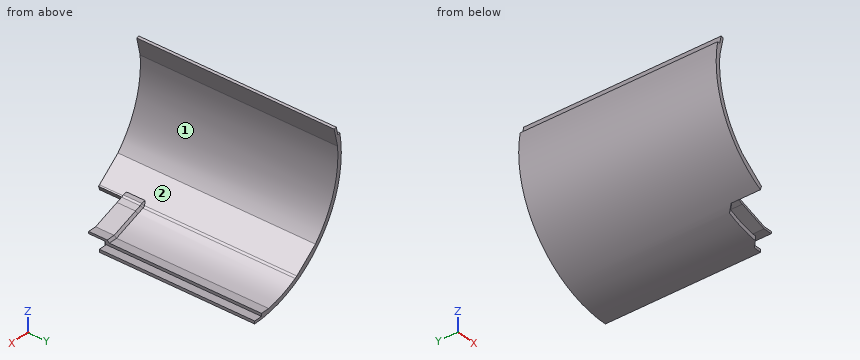
from build123d import *

# Parameters (mm, degrees)
EXTRUDE_1_DEPTH     = 96
CUT_EXTRUDE_1_DEPTH = 115.435602569
CUT_EXTRUDE_2_DEPTH = 125.800902391
EXTRUDE_2_DEPTH     = 10
CHAMFER_1_SIZE      = 1


with BuildPart() as part:
    # Эскиз1 → Бобышка-Вытянуть1 (new body)
    with BuildSketch(Plane(origin=(0, 0, 0), x_dir=(1, 0, 0), z_dir=(0, 1, 0))):
        with BuildLine():
            Line((-46.843090279, -12.726935731), (-48.838961005, -3.96936871))
            ThreePointArc((-48.838961005, -3.96936871), (-46.263287314, 16.146462365), (-35.762915695, 33.496475352))
            Line((-35.762915695, 33.496475352), (-24.862084305, 42.224125379))
            ThreePointArc((-24.862084305, 42.224125379), (-24.343954807, 42.524955783), (-23.822185811, 42.819428571))
            ThreePointArc((-23.822185811, 42.819428571), (-16.269960049, 46.22), (-8.252878286, 48.3))
            Line((-8.252878286, 48.3), (-4, 48.3))
            Line((-4, 48.3), (-4, 49.65))
            Line((-4, 49.65), (0, 49.65))
            Line((0, 49.65), (0, 51))
            ThreePointArc((0, 51), (-39.236846594, 32.580206711), (-50.131159715, -9.373730613))
            Line((-50.131159715, -9.373730613), (-48.950659721, -9.104691807))
            Line((-48.950659721, -9.104691807), (-48.061840279, -13.004691807))
            Line((-48.061840279, -13.004691807), (-46.843090279, -12.726935731))
        make_face()
    extrude(amount=EXTRUDE_1_DEPTH)

    # Эскиз2 → Вырез-Вытянуть1 (cut, through all)
    with BuildSketch(Plane(origin=(-12.717132038, 0, -36.127061224), x_dir=(0.9432653061224487, 0, -0.33204000100247416), z_dir=(0.33204000100247416, 0, 0.9432653061224487))):
        Polygon((8.752878286, 0), (8.752878286, 17.5), (-5.459985067, 17.5), (-8.752878286, 14.207106781), (-8.752878286, 0), (-8.252878286, 0), (8.252878286, 0), align=None)
    extrude(amount=-CUT_EXTRUDE_1_DEPTH, mode=Mode.SUBTRACT)

    # Эскиз3 → Вырез-Вытянуть2 (cut, through all)
    with BuildSketch(Plane.XY.offset(-48.3)):
        Polygon((-3.5, 20), (0, 20), (0, 20.5), (-3.707106781, 20.5), (-6.707106781, 17.5), (-8.752878286, 17.5), (-8.752878286, 0), (-8.252878286, 0), (-8.252878286, 17), (-6.5, 17), align=None)
        Polygon((0, 0), (0, 20), (-3.5, 20), (-6.5, 17), (-8.252878286, 17), (-8.252878286, 0), align=None)
    extrude(amount=-CUT_EXTRUDE_2_DEPTH, mode=Mode.SUBTRACT)

    # Эскиз4 → Бобышка-Вытянуть2 (add)
    with BuildSketch(Plane(origin=(0, 12, 0), x_dir=(1, 0, 0), z_dir=(0, 1, 0))):
        with BuildLine():
            Line((-20.660349892, 42.872283268), (-8.082011241, 47.3))
            Line((-8.082011241, 47.3), (-4, 47.3))
            Line((-4, 47.3), (-4, 48.3))
            Line((-4, 48.3), (-8.252878286, 48.3))
            Line((-8.252878286, 48.3), (-20.992389893, 43.815548574))
            Line((-20.992389893, 43.815548574), (-23.822185811, 42.819428571))
            ThreePointArc((-23.822185811, 42.819428571), (-24.343954807, 42.524955783), (-24.862084305, 42.224125379))
            Line((-24.862084305, 42.224125379), (-26.311602254, 41.063582213))
            Line((-26.311602254, 41.063582213), (-24.354694829, 41.362408534))
            ThreePointArc((-24.354694829, 41.362408534), (-23.883747135, 41.636121611), (-23.409723676, 41.904472761))
            Line((-23.409723676, 41.904472761), (-20.660349892, 42.872283268))
        make_face()
    extrude(amount=EXTRUDE_2_DEPTH)

    # Фаска1
    chamfer_1_edges = [part.edges().sort_by_distance(p)[0] for p in [
        (-25.333148542, 22, -41.212995374),
        (-23.883747135, 22, -41.636121611),
        (-15.745867458, 22, -44.602236381),
        (-6.04100562, 22, -47.3),
    ]]
    chamfer(chamfer_1_edges, length=CHAMFER_1_SIZE - 0.0001)  # a hair under: the kernel refuses the full size


solid = part.part
Part model, mm, in its own coordinate system. Face numbers are marked on the shaded views. Coordinates: 2 decimals unless noted, no trailing zeros. Loops run counter-clockwise (first coordinate to the right, second up) from the corner with the lowest first, then second, coordinate; pieces in that order, holes last. Notation, with made-up numbers: (73.25, 54) -> (96.25, 54) arc R8 cw to (96.25, 66) -> close; hole circle Ø2 at (-8.5, 75). An arc over 180 degrees is marked (long way). Use a Markdown table: item, result. Add a question column.
Item 1: Band-saw the part on B-B on y = 30. Write the cut outline in (x, z).
Item 2: Band-saw the part on C-C on z = 0. Write the cut outline in (x, y).
Item 3: Flat gauge pins, fed straight in: P1, Ø4.5, axis at x = -5.5, y = 18, coming from the +Z side; P2, Ø1.3, axis at x = -5.5, y = 15.5, coming from the -Z side; P3, Ø1.3, axis at x = -7, y = 45, coming from the +Z side. Where does each tip first touch, or does it go through?
Item 4: Probe probe 1 along X at (y, z) = (15, -1); probe 2 along X at (y, z) = (32.5, -37); probe 3 along Z at (x, y) = (-30, 16). List the from-to ranges inside material, lowest first.
Item 5: Pull direction Z, two halves, no side cores. Call the marked faces 1 and 2: +Z half, -Z half, draft (parallel to the pull), parting line (faces both ways), or undercut.
Geometry says:
| question | item | result |
|---|---|---|
| 1 | outline | (-50.13, 9.37) arc R51 ccw to (0, -51) -> (0, -49.65) -> (-4, -49.65) -> (-4, -48.3) -> (-8.25, -48.3) arc R49 cw to (-24.86, -42.22) -> (-35.76, -33.5) arc R49 cw to (-48.84, 3.97) -> (-46.84, 12.73) -> (-48.06, 13) -> (-48.95, 9.1) -> close |
| 2 | outline | (-51, 0) -> (-49, 0) -> (-49, 96) -> (-51, 96) -> close |
| 3 | P1 | z = -47.3 |
| 3 | P2 | z = -48.3 |
| 3 | P3 | z = -48.3 |
| 4 | probe 1 | -50.99 to -48.99 |
| 4 | probe 2 | -35.1 to -31.39 |
| 4 | probe 3 | -41.24 to -38.11 |
| 5 | face 1 | undercut |
| 5 | face 2 | +Z half |
